The drawing under review shows one solid part. Ordinate dimensions are in mm from its lowest x, y, z. A direction names the side the tool comes from. Give positions to 0.01 mm unless a question says otherwise; leave off trailing zeros. Order: outer loops, then holes, each group sorted by start corner. A loop starts at its lowest first (then second) coordinate and runs counter-clockwise, first axis right, second up. Notation, with made-up numbers: (82, 63) -> (115, 63) arc R35 cw to (115, 101) -> close; hole circle Ø2 at (-29.75, 38.5). An arc over 180 degrees is marked (long way). One line per item, written item: value.
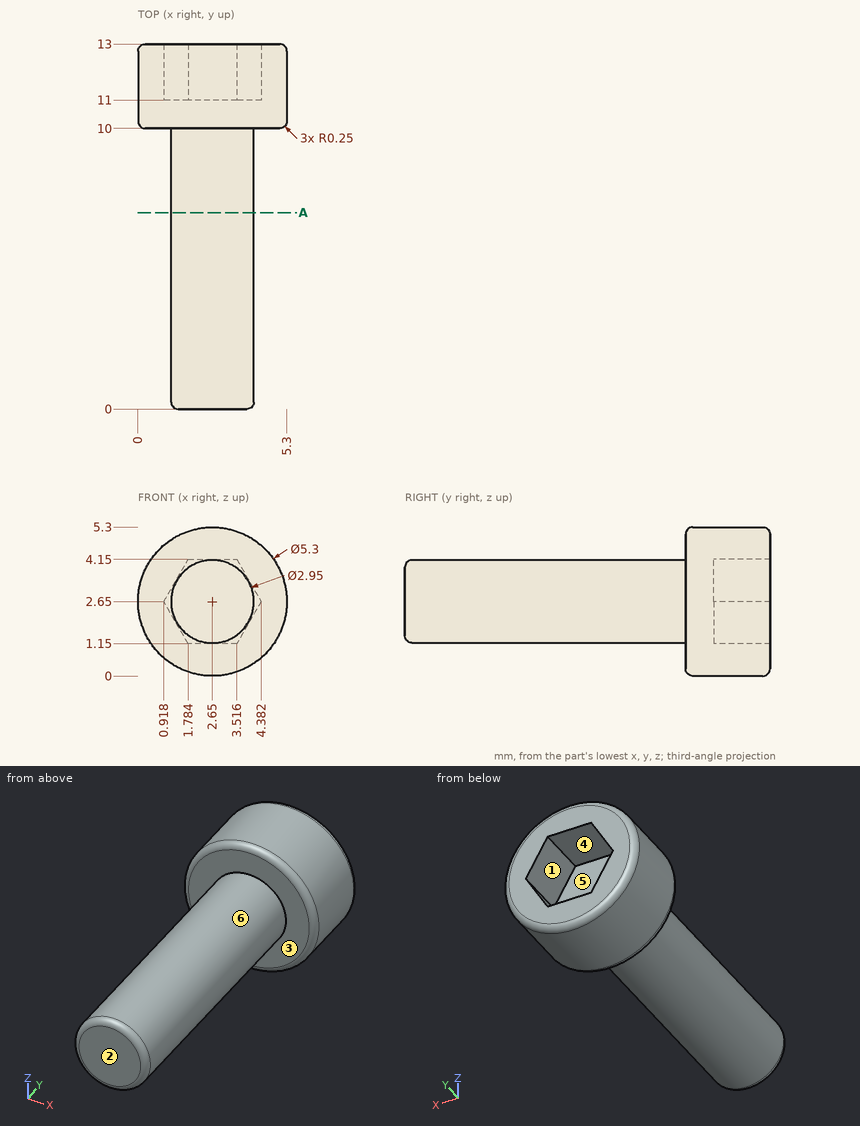
Item 1: To check wall thickness, follow line 1 along Y through (x, z) = (1.75, 4.8); line 2 along Z through (x, y) = (2.7, 5.5); line 3 along Y through (x, z) = (2.95, 3.05). State the ranges of each line that lie inside material, in increasing order. Write a range as from..to.
Returned:
line 1: 10..13
line 2: 1.18..4.12
line 3: 0..11
Item 2: Machinability: for the marked faces 1 and 2, which of the approach directions +Z, -Z, +X, -X, +Y, -Y give a long, thin tool a straight path to every point of the face, cutting with its end or side? Answer none if there is none.
Returned:
face 1: +Y
face 2: +Z, -Z, +X, -X, -Y
Item 3: Clearance check with a flat-ended pin moving along its axis: P1, Ø1, axis at y = 10, z = 2.5, coming from the +X side. State where the tip first meets the part, or that it passes through.
Returned:
P1: x = 5.3
Item 4: Draft analysis for pull direction X (two halves, no side actions). For the marked faces 3, 4, 5 and 6, state which applies: pulls with the +X half, pulls with the -X half, needs draft (parallel to the pull), parting line crosses it, or undercut.
Returned:
face 3: needs draft
face 4: undercut
face 5: undercut
face 6: parting line crosses it
Item 5: Add section A-A on y = 7. Give the boundary of the cut face in (x, z) (3 decimals).
Returned:
outline: circle Ø2.95 at (2.65, 2.65)
